Autodesk Inventor part; units mm, degrees
ref_plane "Work Plane1" through (0, 0, 0) normal (0, 0, 1) x (1, 0, 0)
ref_plane "YZ Plane" through (0, 0, 0) normal (1, 0, 0) x (0, 1, 0)
ref_plane "XZ Plane" through (0, 0, 0) normal (0, 1, 0) x (-1, 0, 0)
ref_plane "Work Plane1" through (0, 0, 0) normal (0, 0, 1) x (1, 0, 0)
sketch "Sketch1" plane through (0, 0, 0) normal (0, 0, 1) x (1, 0, 0)
  circle A0 centre (-4, 62) radius 1.75
  circle A1 centre (-4, 50) radius 1.75
  line L0 (-8, 12) -> (-8, 66)
  line L1 (0, 66) -> (-8, 66)
  line L2 (0, 66) -> (0, 36)
  line L3 (0, 36) -> (-8, 36)
  line L4 (0, 66) -> (0, 91)
  line L5 (0, 91) -> (-4, 91)
  line L6 (-4, 91) -> (-4, 70)
  line L7 (-4, 70) -> (-8, 66)
  line L8 (-8, 66) -> (-8, 36)
  line L9 (-4, 62) -> (-4, 40) construction
  line L10 (-5.75, 62) -> (-5.75, 40)
  line L11 (-2.25, 40) -> (-2.25, 62)
  arc A2 (-2.25, 62) -> (-5.75, 62) centre (-4, 62) ccw
  arc A3 (-5.75, 40) -> (-2.25, 40) centre (-4, 40) ccw
  line L12 (-4, 80.5) -> (0, 80.5) construction
  point P0 (0, 0)
  point P1 (-4, 51)
  point P2 (-2.25, 62)
  dimension "d4" = 21
  dimension "d6" = 4
  dimension "d7" = 135
  dimension "d8" = 30
  dimension "d11" = 4
  dimension "d12" = 22
  dimension "d13" = 1.75
extrude "Extrusion1" add sketch "Sketch1" along normal blind 4
sketch "Sketch2" plane through (0, 0, 4) normal (0, 0, 1) x (1, 0, 0)
  arc A0 (-2.25, 62) -> (-5.75, 62) centre (-4, 62) ccw
  arc A1 (-5.75, 40) -> (-2.25, 40) centre (-4, 40) ccw
  line L0 (-4, 62) -> (-4, 40) construction
  line L1 (-7, 62) -> (-7, 40)
  line L2 (-1, 40) -> (-1, 62)
  arc A2 (-1, 62) -> (-7, 62) centre (-4, 62) ccw
  arc A3 (-7, 40) -> (-1, 40) centre (-4, 40) ccw
  point P0 (0, 0)
  point P1 (-4, 51)
  dimension "d16" = 6
extrude "Extrusion2" cut sketch "Sketch2" against normal blind 1.5
sketch "Sketch3" plane through (0, 0, 4) normal (0, 0, 1) x (1, 0, 0)
  line L0 (0, 36) -> (0, 91)
  line L1 (0, 87.1) -> (-4, 87.1)
  line L2 (-4, 91) -> (-4, 70)
  line L3 (-4, 71) -> (0, 71)
  line L4 (0, 74.9) -> (-4, 74.9)
  line L5 (0, 91) -> (-4, 91)
  point P0 (0, 0)
  point P1 (0, 70)
  dimension "d19" = 3.9
  dimension "d20" = 3.9
  dimension "d30" = 1
extrude "Extrusion3" add sketch "Sketch3" along normal blind 4.2 contours L3 L2 L4 L0 | L1 L2 L5 L0
sketch "Sketch4" plane through (-4, 91, 0) normal (0, 1, 0) x (1, 0, 0)
  circle A0 centre (2, -6.2) radius 1
  line L0 (4, -8.2) -> (0, -8.2)
  point P0 (4, 0)
  point P1 (2, -8.2)
  dimension "d23" = 2
  dimension "d24" = 2
extrude "Extrusion4" cut sketch "Sketch4" against normal up to surface (3.9 mm away)
sketch "Sketch5" plane through (-4, 71, 4) normal (0, -1, 0) x (1, 0, 0)
  circle A0 centre (2, 2.2) radius 1
  circle A1 centre (2, 2.2) radius 1.2
  point P0 (4, -4)
  dimension "d27" = 2.4
extrude "Extrusion5" cut sketch "Sketch5" against normal up to surface (3.9 mm away) contours A0 | A1
fillet "Fillet1" radius 2.4 1 edges at (-4, 70, 2)
fillet "Fillet2" radius 4 2 edges at (-8, 36, 2) (0, 36, 2)
fillet "Fillet3" radius 8 1 edges at (-8, 66, 2)
fillet "Fillet4" radius 0.5 25 edges at (0, 91, 4.1) (-4, 91, 4.1) (-2, 91, 0) (-6.8286, 37.1714, 0) (-8, 51.3429, 0) (-7.391, 65.7478, 0) (-5.1799, 68.8201, 0) (-4.1827, 70.0757, 0) (-4, 80.9971, 0) (0, 65.4998, 0) (-4, 89.05, 8.2) (-2, 91, 8.2) (0, 89.05, 8.2) (-4, 71, 6.1) (0, 71, 6.1) (-2, 71, 8.2) (-4, 72.95, 8.2) (0, 72.95, 8.2) (-5.1799, 68.8201, 4) (-4.1827, 70.0757, 4) (-4, 70.9971, 4) (-8, 51.3429, 4) (-6.8286, 37.1714, 4) (0, 55.4998, 4) (-7.391, 65.7478, 4)
sketch "Sketch6" plane through (0, 0, 4) normal (0, 0, 1) x (1, 0, 0)
  line L0 (-4, 87.1) -> (-4, 74.9)
  line L1 (-4, 81) -> (0, 81) construction
  arc A0 (-2.25, 62) -> (-5.75, 62) centre (-4, 62) ccw
  line L2 (-4, 62) -> (-4, 61)
  point P0 (0, 0)
  dimension "d35" = 1
  dimension "d36" = 20
properties part number "wiperholder"
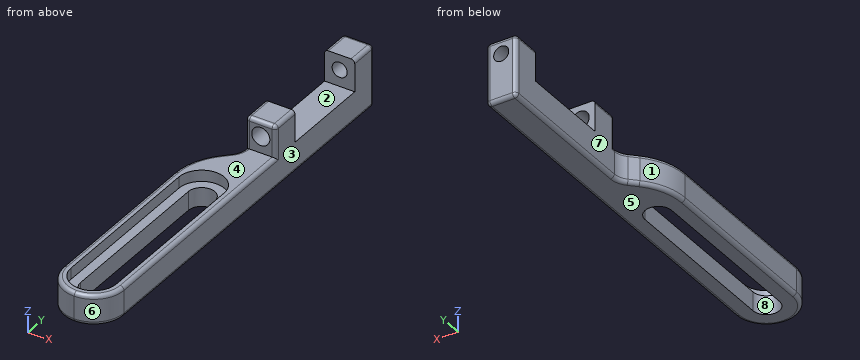
CAD build for the part. Positions are in the model's coordinates, mm. Face numbers are marked on the shaded views. A direction names the side the tool comes from. Give positions to 0.01 mm unless a question says otherwise; leave off trailing zeros. Order: outer loops, then holes, each group sorted by start corner. A loop starts at its lowest first (then second) coordinate and runs counter-clockwise, first axis right, second up.
(1) Saw through at A-A, the plane z = 6.2. Give the cut face in (x, y).
(2) Drill centre lines: L1, parallel to Y at x = -1.75, z = 4.25; L2, parallel to X at y = 89.3, z = 6.2; L3, parallel to Z at x = -2, y = 89.9. Where is each one in solid material? Low to high.
(3) Saw through at D-D, the plane y = 83. Give the cut face in (x, z).
(4) Tool access for the marked faces 4, 5, 6, 7 and 8: list every direction of +Z, -Z, +X, -X, +Y, -Y with a clear straight run to the whole face (end or side of a thin tool).
(5) Flat gauge pins, fed straight in: pin 1 (1.2 mm diameter, centred on x = -2.5, y = 83, fed in from +Z); pin 2 (3.5 mm diameter, centred on x = -2.5, z = 5, fed in from -Y) (3 decimals); pin 3 (3.5 mm diameter, centred on x = -4.5, y = 53, fed in from +Z). Where does each tip first touch, or does it go through?
(6) Saw through at B-B, the plane y = 45.5. Give the cut face in (x, z), then the cut area to 3 significant figures.
(7) Mould opens along Y. For the marked faces 1, 2 and 3 say: released by +Y, released by -Y, zero draft, split by the parting line, or undercut.
Results found:
1. outline: (-4, 71.5) arc R0.5 ccw to (-3.5, 71) - (-3.2, 71) - (-3.2, 74.9) - (-4, 74.9) - close; (-4, 87.1) - (-3, 87.1) - (-3, 91) - (-3.5, 91) arc R0.5 ccw to (-4, 90.5) - close; (-1, 87.1) - (0, 87.1) - (0, 90.5) arc R0.5 ccw to (-0.5, 91) - (-1, 91) - close; (-0.8, 71) - (-0.5, 71) arc R0.5 ccw to (0, 71.5) - (0, 74.9) - (-0.8, 74.9) - close
2. L1: y = 71 to 74.9, 87.1 to 91
2. L2: x = -4 to -3, -1 to 0
2. L3: z = 0 to 5.2, 7.2 to 8.2
3. outline: (-4, 0.5) arc R0.5 ccw to (-3.5, 0) - (-0.5, 0) arc R0.5 ccw to (0, 0.5) - (0, 4) - (-4, 4) - close
4. face 4: +Z, +X, -X, -Y
4. face 5: -Z, +X, -X, +Y, -Y
4. face 6: +Z, -Z, +X, -Y
4. face 7: +Z, -Z, -X, +Y
4. face 8: +Z, -Z
5. pin 1: stops at z = 4
5. pin 2: stops at y = 36.035
5. pin 3: stops at z = 2.5
6. outline: (-8, 0.5) arc R0.5 ccw to (-7.5, 0) - (-5.75, 0) - (-5.75, 2.5) - (-7, 2.5) - (-7, 4) - (-7.5, 4) arc R0.5 ccw to (-8, 3.5) - close; (-2.25, 0) - (-0.5, 0) arc R0.5 ccw to (0, 0.5) - (0, 3.5) arc R0.5 ccw to (-0.5, 4) - (-1, 4) - (-1, 2.5) - (-2.25, 2.5) - close
6. area: 14.0 mm2
7. face 1: released by +Y
7. face 2: undercut
7. face 3: zero draft
